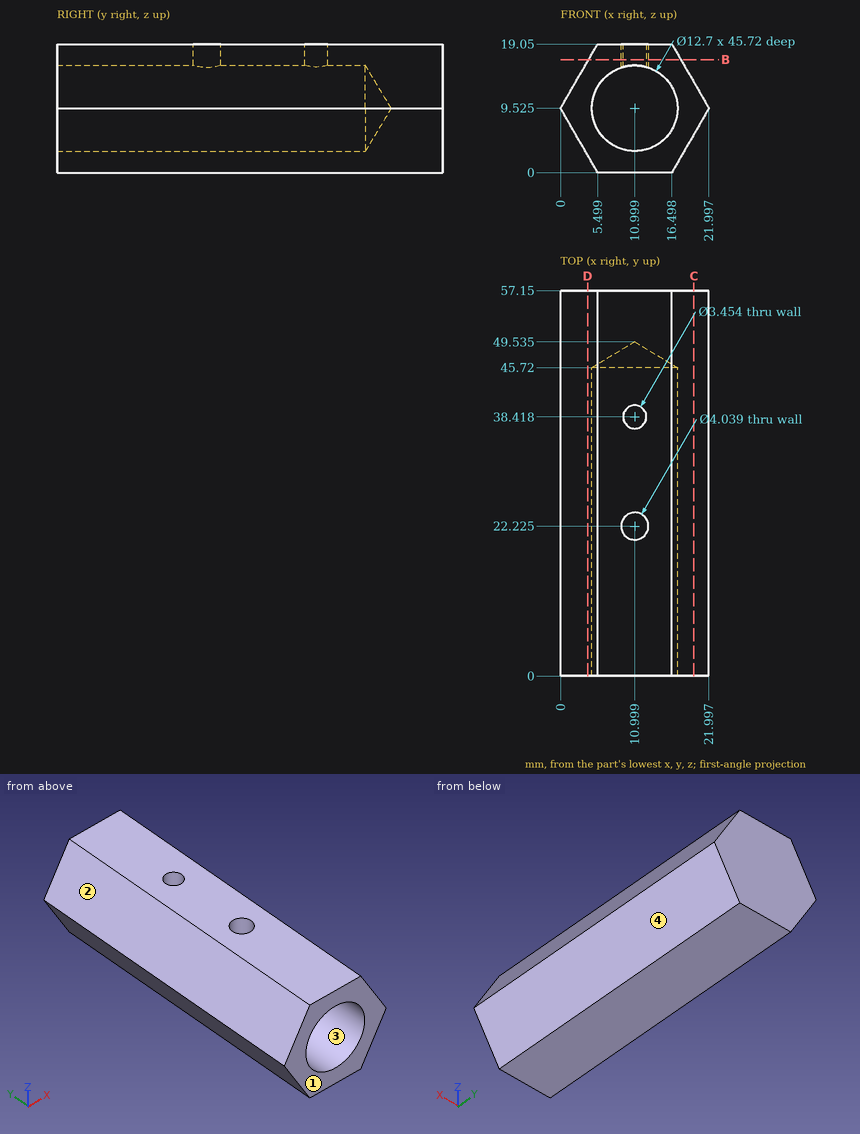
Input: dimensioned drawing with shaded views. Units: mm. Origin: part minimum x, y, z. Round coordinates to 2 decimals unless told otherwise and drop trailing zeros. Order: outer loops, then holes, each group sorted by start corner. A loop starts at its lowest first (then second) coordinate and runs counter-clockwise, first axis right, second up. Notation, with made-up numbers: (12.25, 54.5) - (39.25, 54.5) arc R11 ccw to (39.25, 68.5) - close; hole circle Ø2 at (-29, 20). An arc over 180 degrees is marked (long way). Answer as a JSON object with one key per item and string values. Group by question number.
(1) Draft query along Z for the marked faces 1, 2, 3 and 4. Return one class per face: released by +Z, released by -Z, zero draft, split by the parting line, or undercut.
(2) Cut plane C-C (x = 19.75). Return loops of the section in (y, z).
(3) Cut plane B-B (z = 16.75). Count the separate pieces of the cut face and the enclosed holes in it, then the cut area to 3 significant figures.
(4) Material intervals for probe 1 along X at (y, z) = (15.5, 5.75) (1 decimal); probe 2 along X at (y, z) = (31.5, 8) (1 decimal); probe 3 along Z at (x, y) = (11.25, 43), sorted ascending. Write a range as from..to.
(5) Pin query (flat end, axial travel): P1, Ø1, axis at x = 19.5, y = 31.5, coming from the -Z side (1 decimal); P2, Ø5, axis at y = 42, z = 4.5, coming from the +X side. Return the tip coordinate at first contact, or that it passes through.
(6) Cut plane D-D (x = 4). Return loops of the section in (y, z), then the cut area to 3 significant figures.
Here are the results:
{
 "1": {"face 1": "zero draft", "face 2": "released by +Z", "face 3": "undercut", "face 4": "released by -Z"},
 "2": {"outline": "(0, 5.63) - (57.15, 5.63) - (57.15, 13.42) - (0, 13.42) - close"},
 "3": {"separate pieces": "1", "enclosed holes": "2", "area": "758 mm^2"},
 "4": {"probe 1": "x = 2.2..5.9, 16.1..19.8", "probe 2": "x = 0.9..4.8, 17.2..21.1", "probe 3": "z = 0..3.18, 15.87..19.05"},
 "5": {"P1": "stops at z = 4.3", "P2": "stops at x = 20.54"},
 "6": {"outline": "(0, 2.6) - (57.15, 2.6) - (57.15, 16.45) - (0, 16.45) - close", "area": "792 mm^2"}
}
